```python
from build123d import *

# Parameters (mm, degrees)
F1_DEPTH = 3.175
F2_F1_R  = 2.54
F2_F2_R  = 2.54


with BuildPart() as f1:
    # F0 (on Front) → F1 (new body, symmetric)
    with BuildSketch(Plane.XZ):
        with BuildLine():
            Line((13.3350007236, 17.7493449301), (-3.0348624568, 17.7493449301))
            Line((-3.0348624568, 17.7493449301), (-3.0348624568, 8.3688618615))
            ThreePointArc((-3.0348624568, 8.3688618615), (7.007326367, 9.8180073261), (13.3350007236, 17.7493449301))
        make_face()
        Polygon((-3.0348624568, 8.3688618615), (-3.0348624568, 17.7493449301), (-8.8243288919, 17.7493449301), (-8.8243288919, -4.8698359169), (-3.0348624568, -4.6902415343), align=None)
    extrude(amount=F1_DEPTH, both=True)

    # F2: fillet of radius 2.54 on 4 edges, made by hand

    # F2_f1
    f2_f1_edges = [f1.edges().sort_by_distance(p)[0] for p in [
        (-3.0348624568, 0, 8.3688618615),
    ]]
    fillet(f2_f1_edges, radius=F2_F1_R)

    # F2_f2
    f2_f2_edges = [f1.edges().sort_by_distance(p)[0] for p in [
        (-3.0348624568, 3.175, 0.3884883664),
        (-3.0348624568, -3.175, 0.3884883664),
        (-3.0348624568, 0, -4.6902415343),
        (-2.2547093843, -3.175, 7.2987582727),
        (-2.2547093843, 3.175, 7.2987582727),
    ]]
    fillet(f2_f2_edges, radius=F2_F2_R)


solid = f1.part
```
CAD build for the part. Positions are in the model's coordinates, mm. A direction names the side the tool comes from. Round coordinates to 2 decimals unless told otherwise and drop trailing zeros. Write each loop counter-clockwise with the first axis right and the second up, starting at its lowest first coordinate (ties: lowest second). Pieces come first, ordered by that corner, then holes. Notation, with made-up numbers: (36, 42.5) -> (66, 42.5) arc R21 cw to (66, 70.5) -> close; hole circle Ø3 at (53.25, 88). An arc over 180 degrees is marked (long way). Answer in a Markdown table with one row per item. Add a question column.
Item 1: Drop flat-ended pins along their axis: pin 1 Ø3 at (y, z) = (-1.5, 15) entering from +X; pin 2 Ø1 at (x, z) = (-2, 2) entering from -Y. Give the stop position or say it passes through.
Item 2: Drill centre lines: line 1 (Z direction, x = -5.5, y = 2.5); line 2 (X direction, y = 0.5, z = 1.5); line 3 (Z direction, x = 10, y = 2.5). Where is each one in solid material? Low to high. Write a range as from..to.
Item 3: Saw through at B-B, the plane y = 2.75. Write the cut outline in (x, z), then the cut area to 3 significant figures.
Item 4: Saw through at A-A, the plane z = -0.75. Write the cut outline in (x, y) (3 decimals).
Item 5: Which spindle directions (+Z, -Z, +X, -X, +Y, -Y) get a long thin tool onto all of the face, cutting with end or side? Do faces 1 (the face through (-3.8, -2.45, 0.42)), 2 (the face through (2, 0, 17.749)), 3 (the face through (-4, -3.175, 12)), 4 (the face through (-3.035, 0, 2)), 5 (the face through (-3.8, 2.45, 0.42)). Say none if no direction does.
Findings below:
| question | item | result |
|---|---|---|
| 1 | pin 1 | stops at x = 12.82 |
| 1 | pin 2 | passes through |
| 2 | line 1 | z = -4.77..17.75 |
| 2 | line 2 | x = -8.82..-3.03 |
| 2 | line 3 | z = 13.34..17.75 |
| 3 | outline | (-8.82, -4.87) -> (-5.5, -4.77) arc R2.54 ccw to (-4.17, -4.34) -> (-4.17, 5.47) arc R3.67 cw to (-0.35, 9.14) arc R12.65 ccw to (12.14, 17.75) -> (-8.82, 17.75) -> close |
| 3 | area | 221 mm^2 |
| 4 | outline | (-8.824, -3.175) -> (-5.575, -3.175) arc R2.54 ccw to (-3.035, -0.635) -> (-3.035, 0.635) arc R2.54 ccw to (-5.575, 3.175) -> (-8.824, 3.175) -> close |
| 5 | face 1 | -Z, +X, -Y |
| 5 | face 2 | +Z, +X, -X, +Y, -Y |
| 5 | face 3 | +Z, -Z, +X, -X, -Y |
| 5 | face 4 | -Z, +X, +Y, -Y |
| 5 | face 5 | -Z, +X, +Y |
